Read the model definition and answer for the solid it produces. Units are mm, in the model's axes. Face numbers are marked on the shaded views. A direction names the side the tool comes from. Coordinates: 2 decimals unless noted, no trailing zeros. Write each loop counter-clockwise with the first axis right and the second up, starting at its lowest first coordinate (ties: lowest second). Pieces come first, ordered by that corner, then holes.
(1) The mould has two halves that part along Z. Classify the marked faces 4, 5 and 6: +Z half, -Z half, draft (parallel to the pull), parting line (faces both ways), or undercut.
(2) Given pin 1 (2 mm diameter, centred on x = -12.5, z = 4, fed in from -Y); pin 2 (16.5 mm diameter, centred on x = 4.5, z = -10, fed in from +Y); pin 3 (10 mm diameter, centred on x = 43, z = 89, fed in from +Y); pin 4 (12 mm diameter, centred on x = -7, y = 24, fed in from +Z), each flat-ended and moving along its own axis, determine where each tip first touches the part or whether it passes through.
(3) Which of the six approach directions +Z, -Z, +X, -X, +Y, -Y give full straight-line access (tool end or side, diameter ignored) to the marked faces 1, 2 and 3?
(4) Find the intervals of material crossed by probe 1 along Z at (x, y) = (38.5, 19.75); probe 2 along Z at (x, y) = (38.5, 37.5); probe 3 along Z at (x, y) = (-52, 2), in increasing order.
(5) Section D-D on x = -39.5 is taken. Write down the section's boundary in (y, z), then the cut area to 3 significant figures.
(6) Section B-B on z = -2.5 is taken. Write down the section's boundary in (x, y).
(7) Section A-A on y = 0 is taken. Write down the section's boundary in (x, z), then the cut area to 3 significant figures.
(8) Section C-C on x = -7 is taken. Write down the section's boundary in (y, z), then the cut area to 3 significant figures.
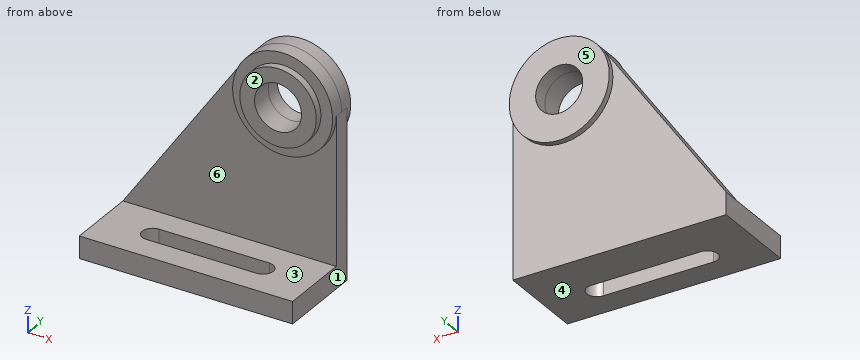
from build123d import *

# Parameters (mm, degrees)
F0_W     = 145
F0_H     = 12
F1_DEPTH = 15
F4_DEPTH = 12
F6_R     = 26
F6_R_2   = 16
F7_DEPTH = 10
F8_DEPTH = 10
F9_DEPTH = 15


with BuildPart() as f1:
    # F0 (on Top) → F1 (new body)
    with BuildSketch(Plane.XY):
        with Locations((0, 30)):
            Rectangle(F0_W, F0_H)
        Polygon((-72.5, 24), (-72.5, 0), (-72.5, -24), (-37.5, -24), (37.5, -24), (72.5, -24), (72.5, 0), (72.5, 24), align=None)
        with BuildLine():
            Line((37.5, -7), (-37.5, -7))
            ThreePointArc((-37.5, -7), (-44.5, 0), (-37.5, 7))
            Line((-37.5, 7), (37.5, 7))
            ThreePointArc((37.5, 7), (44.5, 0), (37.5, -7))
        make_face(mode=Mode.SUBTRACT)
    extrude(amount=-F1_DEPTH)

    # F3 (on offset) → F4 (join)
    with BuildSketch(Plane(origin=(0, 36, 0), x_dir=(-1, 0, 0), z_dir=(0, 1, 0))):
        with BuildLine():
            ThreePointArc((-10.5910955607, 119.4188839277), (-6.0584930148, 110.1758844594), (-4.5, 100))
            ThreePointArc((-4.5, 100), (-38.5, 66), (-72.5, 100))
            Line((-72.5, 100), (-72.5, 0))
            Line((-72.5, 0), (72.5, 0))
            Line((72.5, 0), (-10.5910955607, 119.4188839277))
        make_face()
    extrude(amount=-F4_DEPTH)

    # F6 (on offset) → F7 (join)
    with BuildSketch(Plane(origin=(0, 30, 0), x_dir=(-1, 0, 0), z_dir=(0, 1, 0))):
        with BuildLine():
            ThreePointArc((-72.5, 100), (-38.5, 66), (-4.5, 100))
            ThreePointArc((-4.5, 100), (-38.5, 134), (-72.5, 100))
        make_face()
        with Locations((-38.5, 100)):
            Circle(F6_R, mode=Mode.SUBTRACT)
        with Locations((-38.5, 100)):
            Circle(F6_R)
        with Locations((-38.5, 100)):
            Circle(F6_R_2, mode=Mode.SUBTRACT)
    extrude(amount=F7_DEPTH)

    # F6 (on offset) → F8 (join)
    with BuildSketch(Plane(origin=(0, 30, 0), x_dir=(-1, 0, 0), z_dir=(0, 1, 0))):
        with BuildLine():
            ThreePointArc((-72.5, 100), (-38.5, 66), (-4.5, 100))
            ThreePointArc((-4.5, 100), (-38.5, 134), (-72.5, 100))
        make_face()
        with Locations((-38.5, 100)):
            Circle(F6_R, mode=Mode.SUBTRACT)
    extrude(amount=-F8_DEPTH)

    # F6 (on offset) → F9 (join)
    with BuildSketch(Plane(origin=(0, 30, 0), x_dir=(-1, 0, 0), z_dir=(0, 1, 0))):
        with Locations((-38.5, 100)):
            Circle(F6_R)
        with Locations((-38.5, 100)):
            Circle(F6_R_2, mode=Mode.SUBTRACT)
    extrude(amount=-F9_DEPTH)


solid = f1.part
Response:
1. face 4: -Z half
1. face 5: draft
1. face 6: undercut
2. pin 1: stops at y = 24
2. pin 2: stops at y = 36
2. pin 3: stops at y = 40
2. pin 4: stops at z = 102.76
3. face 1: +Z, -Z, +X, +Y, -Y
3. face 2: +Z, +X, -X, -Y
3. face 3: +X, -X, -Y
4. probe 1: z = -15 to 0, 74 to 84, 116 to 126
4. probe 2: z = 66 to 84, 116 to 134
4. probe 3: z = -15 to 0
5. outline: (-24, -15) - (-6.71, -15) - (-6.71, 0) - (-24, 0) - close; (6.71, -15) - (36, -15) - (36, 47.43) - (24, 47.43) - (24, 0) - (6.71, 0) - close
5. area: 1,270 mm2
6. outline: (-72.5, -24) - (72.5, -24) - (72.5, 36) - (-72.5, 36) - close; hole (-37.5, -7) - (37.5, -7) arc R7 ccw to (37.5, 7) - (-37.5, 7) arc R7 ccw to start
7. outline: (-72.5, -15) - (-44.5, -15) - (-44.5, 0) - (-72.5, 0) - close; (44.5, -15) - (72.5, -15) - (72.5, 0) - (44.5, 0) - close
7. area: 840 mm2
8. outline: (-24, -15) - (-7, -15) - (-7, 0) - (-24, 0) - close; (7, -15) - (36, -15) - (36, 94.14) - (24, 94.14) - (24, 0) - (7, 0) - close
8. area: 1,820 mm2
